Could you check a few things on this model? Use its own coordinates, in mm. A direction names the side the tool comes from. Give positions to 0.01 mm unless a question says otherwise; leave off trailing zeros. Loops run counter-clockwise (first coordinate to the right, second up) from the corner with the lowest first, then second, coordinate; pieces in that order, holes last.
1. I need wall thicknesses on line 1 along X through (y, z) = (2.1, -15); line 2 along Y through (x, z) = (10, 3.3); line 3 along Y through (x, z) = (20, 2). Which ranges of each line are inside material? Lowest first, please.
2. Imagine slicing it at B-B (x = 45). List the corners of the cut face in (y, z) for me.
3. For P1, Ø8, axis at y = 19, z = -6.5, coming from the -X side (3 decimals); P2, Ø7, axis at x = 25, z = -15, coming from the -Y side; P3, Ø7, axis at x = 10, y = 6.25, coming from the -Z side; P4, Ø7, axis at x = 45, z = -15, coming from the +Y side, each with a flat end and sliding along its axis, tell me the tip position at first contact or that it passes through.
4. Imagine slicing it at C-C (z = -15). List the corners of the cut face in (x, y) for me.
5. For faces 5 (the flat face through (35, 5, -16)), 6 (the flat face through (0, 12, 2)), 7 (the flat face through (20, 3, -13)), which set-ups out of +Z, -Z, +X, -X, +Y, -Y let a thin tool reach every point of the face, with its end or its side?
6. Imagine slicing it at A-A (y = 18.75). List the corners of the cut face in (x, z) for me, plus the area to 4 significant figures.
7. Thinking about a two-plate mould opening in Y: for faces 1 (the flat face through (25, 25, 2)), 2 (the flat face through (30, 0, -6)), 3 (the cylindrical face through (21.586, 10.013, 2.241)), 4 (the flat face through (19.1, 15.5, 0)), which applies, +Y half, -Y half, draft (parallel to the pull), parting line (faces both ways), or undercut?
8. Imagine slicing it at D-D (x = 38). List the corners of the cut face in (y, z) for me.
```python
from build123d import *

# Parameters (mm, degrees)
CROQUIS1_W              = 50
CROQUIS1_H              = 25
CROQUIS1_R              = 2.95
SALIENTE_EXTRUIR1_DEPTH = 5
CROQUIS2_W              = 30
CROQUIS2_H              = 25
CROQUIS2_R              = 3
SALIENTE_EXTRUIR2_DEPTH = 5
REDONDEO1_R             = 7


with BuildPart() as part:
    # Croquis1 → Saliente-Extruir1 (new body)
    with BuildSketch(Plane.XY):
        with Locations((25, 12.5)):
            Rectangle(CROQUIS1_W, CROQUIS1_H)
        with Locations((10, 18.75)):
            Circle(CROQUIS1_R, mode=Mode.SUBTRACT)
        with Locations((10, 6.25)):
            Circle(CROQUIS1_R, mode=Mode.SUBTRACT)
        with Locations((20, 12.5)):
            Circle(CROQUIS1_R, mode=Mode.SUBTRACT)
    extrude(amount=SALIENTE_EXTRUIR1_DEPTH)

    # Croquis2 → Saliente-Extruir2 (add)
    with BuildSketch(Plane.XZ):
        with Locations((35, -12.5)):
            Rectangle(CROQUIS2_W, CROQUIS2_H)
        with Locations(Location((45, -15, 0), (0, 0, 270))):
            Circle(CROQUIS2_R, mode=Mode.SUBTRACT)
        with Locations(Location((25, -15, 0), (0, 0, 270))):
            Circle(CROQUIS2_R, mode=Mode.SUBTRACT)
    extrude(amount=-SALIENTE_EXTRUIR2_DEPTH)

    # Redondeo1
    # the kernel refuses this fillet: 7 mm, written as the material it adds along each edge
    with BuildSketch(Plane(origin=(20, 5, 0), x_dir=(0, 0, -1), z_dir=(1, 0, 0))) as redondeo1_piece_1_section:
        with BuildLine():
            CenterArc((REDONDEO1_R, REDONDEO1_R), REDONDEO1_R, 180, 90)
            Line((0, REDONDEO1_R), (0, 0))
            Line((0, 0), (REDONDEO1_R, 0))
        make_face()
    redondeo1_piece_1 = extrude(amount=30, mode=Mode.PRIVATE)
    redondeo1_piece_1 = redondeo1_piece_1 - Plane(origin=(20, 12.5, -1.59035859), x_dir=(1, 0, 0), z_dir=(0, 0, -1)) * Cylinder(2.95, 88, mode=Mode.PRIVATE)
    add(redondeo1_piece_1)


solid = part.part
```
Derived:
1. line 1: x = 20 to 22, 28 to 42, 48 to 50
1. line 2: y = 0 to 3.3, 9.2 to 15.8, 21.7 to 25
1. line 3: y = 0 to 9.55, 15.45 to 25
2. outline: (0, -25) - (5, -25) - (5, -18) - (0, -18) - close; (0, -12) - (5, -12) - (5, -7) arc R7 cw to (12, 0) - (25, 0) - (25, 5) - (0, 5) - close
3. P1: passes through
3. P2: stops at y = 0
3. P3: stops at z = 0
3. P4: stops at y = 5
4. outline: (20, 0) - (22, 0) - (22, 5) - (20, 5) - close; (28, 0) - (42, 0) - (42, 5) - (28, 5) - close; (48, 0) - (50, 0) - (50, 5) - (48, 5) - close
5. face 5: -Z, +X, -X, +Y
5. face 6: +Z, -Z, -X, +Y, -Y
5. face 7: -Z, -X, +Y, -Y
6. outline: (0, 0) - (7.05, 0) - (7.05, 5) - (0, 5) - close; (12.95, 0) - (50, 0) - (50, 5) - (12.95, 5) - close
6. area: 220.5 mm2
7. face 1: +Y half
7. face 2: -Y half
7. face 3: undercut
7. face 4: draft
8. outline: (0, -25) - (5, -25) - (5, -7) arc R7 cw to (12, 0) - (25, 0) - (25, 5) - (0, 5) - close
